from build123d import *

# Parameters (mm, degrees)
SKETCH1_W                          = 36
SKETCH1_H                          = 68
BOSS_EXTRUDE1_DEPTH                = 15
F_1_16_0_116_DOWEL_HOLE1_OUTLINE_R = 1.4732
F_1_16_0_116_DOWEL_HOLE1_DEPTH     = 15
SKETCH5_R                          = 3.175
BOSS_EXTRUDE2_DEPTH                = 7.62


# Read off the part's stored shape, not the designer's step: 1/16 (0.116) Dowel Hole1
with BuildPart() as part:
    # Sketch1 → Boss-Extrude1 (new body)
    with BuildSketch(Plane.XY):
        Rectangle(SKETCH1_W, SKETCH1_H)
    extrude(amount=BOSS_EXTRUDE1_DEPTH)

    # 1/16 (0.116) Dowel Hole1 outline → 1/16 (0.116) Dowel Hole1 (cut)
    with BuildSketch(Plane.XY):
        with Locations((15.25, 31.206)):
            Circle(F_1_16_0_116_DOWEL_HOLE1_OUTLINE_R)
        with Locations((-15.25, 0.706)):
            Circle(F_1_16_0_116_DOWEL_HOLE1_OUTLINE_R)
        with Locations((15.25, 0.706)):
            Circle(F_1_16_0_116_DOWEL_HOLE1_OUTLINE_R)
        with Locations((-15.25, 31.206)):
            Circle(F_1_16_0_116_DOWEL_HOLE1_OUTLINE_R)
    extrude(amount=F_1_16_0_116_DOWEL_HOLE1_DEPTH, mode=Mode.SUBTRACT)

    # Sketch5 → Boss-Extrude2 (add)
    with BuildSketch(Plane(origin=(0, 34, 0), x_dir=(1, 0, 0), z_dir=(0, 1, 0))):
        with Locations((0, -7.5)):
            Circle(SKETCH5_R)
    extrude(amount=BOSS_EXTRUDE2_DEPTH)


solid = part.part
Source: CAD feature listing. Evaluate the final solid. Frame: model axes, mm. Round coordinates to 2 decimals unless told otherwise and drop trailing zeros. Order: outer loops, then holes, each group sorted by start corner. A loop starts at its lowest first (then second) coordinate and runs counter-clockwise, first axis right, second up. Notation, with made-up numbers: (28, 1.25) -> (44, 1.25) arc R18 ccw to (44, 17.25) -> close; hole circle Ø11 at (82.5, 45.25). An arc over 180 degrees is marked (long way). Answer as CSV lines item,"result".
Item 1: Line query: L1, parallel to Y at x = -15.25, z = 3.25; L2, parallel to Y at x = 15.5, z = 4.25; L3, parallel to Y at x = 5, z = 9.5. Output: solid intervals per line, ascending.
A:
L1,"-34 to -0.77, 2.18 to 29.73, 32.68 to 34"
L2,"-34 to -0.75, 2.16 to 29.75, 32.66 to 34"
L3,"-34 to 34"
Item 2: Pull-direction query (X, two-part tool) for faces 1 (the face through (0, 41.62, 7)), 2 (the face through (1.5, 37.8, 10.3)), 3 (the face through (16.655, 1.149, 7.395)); classes: pulls with the +X half, pulls with the -X half, needs draft (parallel to the pull), parting line crosses it, or undercut.
A:
face 1,"needs draft"
face 2,"parting line crosses it"
face 3,"undercut"
Item 3: Section B-B, the plane z = 6.75. Return loops of the section in (x, y).
A:
outline,"(-18, -34) -> (18, -34) -> (18, 34) -> (3.09, 34) -> (3.09, 41.62) -> (-3.09, 41.62) -> (-3.09, 34) -> (-18, 34) -> close; hole circle Ø2.95 at (-15.25, 0.71); hole circle Ø2.95 at (-15.25, 31.21); hole circle Ø2.95 at (15.25, 0.71); hole circle Ø2.95 at (15.25, 31.21)"
Item 4: Section D-D, the plane y = 36. Return loops of the section in (x, z) (3 decimals), plus the area to 3 significant figures.
A:
outline,"circle Ø6.35 at (0, 7.5)"
area,"31.7 mm²"
Item 5: Section C-C, the plane x = 0. Return loops of the section in (y, z) (3 decimals).
A:
outline,"(-34, 0) -> (34, 0) -> (34, 4.325) -> (41.62, 4.325) -> (41.62, 10.675) -> (34, 10.675) -> (34, 15) -> (-34, 15) -> close"
Item 6: Pin query (flat end, axial travel): pin 1 Ø3 at (x, z) = (-7, 13.5) entering from +Y. Return the tip coordinate at first contact, or that it passes through.
A:
pin 1,"y = 34"
Item 7: Section A-A, the plane x = -15.25. Return loops of the section in (y, z).
A:
outline,"(-34, 0) -> (-0.77, 0) -> (-0.77, 15) -> (-34, 15) -> close; (2.18, 0) -> (29.73, 0) -> (29.73, 15) -> (2.18, 15) -> close; (32.68, 0) -> (34, 0) -> (34, 15) -> (32.68, 15) -> close"
